from build123d import *

# Parameters (mm, degrees)
SKETCH1_W           = 40
SKETCH1_H           = 28.8
BOSS_EXTRUDE1_DEPTH = 11
CHAMFER2_SIZE       = 8
CHAMFER2_SIZE2      = 18
SKETCH10_W          = 13.5
SKETCH10_H          = 18.8
CUT_EXTRUDE7_DEPTH  = 6
FILLET1_R           = 1.5
SKETCH11_W          = 40
SKETCH11_H          = 3
CUT_EXTRUDE8_DEPTH  = 8
CUT_EXTRUDE9_DEPTH  = 18.8
CUT_EXTRUDE10_DEPTH = 11
CUT_EXTRUDE2_DEPTH  = 30
SKETCH2_R           = 1.65
CUT_EXTRUDE1_DEPTH  = 12
CUT_EXTRUDE4_DEPTH  = 9
SKETCH15_R          = 3.25
CUT_EXTRUDE12_DEPTH = 1
CUT_EXTRUDE13_DEPTH = 6
CHAMFER4_SIZE       = 3
CHAMFER4_SIZE2      = 5
CHAMFER5_SIZE       = 5
CHAMFER5_SIZE2      = 3
CUT_EXTRUDE11_DEPTH = 9.4
CHAMFER8_SIZE       = 1


with BuildPart() as part:
    # Sketch1 → Boss-Extrude1 (new body)
    with BuildSketch(Plane.XY):
        with Locations((0, 14.4)):
            Rectangle(SKETCH1_W, SKETCH1_H)
    extrude(amount=BOSS_EXTRUDE1_DEPTH)

    # Chamfer2
    chamfer2_edges = [part.edges().sort_by_distance(p)[0] for p in [
        (0, 28.8, 11),
    ]]
    chamfer2_side = [part.faces().sort_by_distance(p)[0] for p in [
        (0, 28.8, 5.5),
    ]]
    chamfer(chamfer2_edges, length=CHAMFER2_SIZE, length2=CHAMFER2_SIZE2, reference=chamfer2_side[0])

    # Sketch10 → Cut-Extrude7 (cut)
    with BuildSketch(Plane.XY.offset(11)):
        with Locations((-13.25, 19.4)):
            Rectangle(SKETCH10_W, SKETCH10_H)
        with Locations((13.25, 19.4)):
            Rectangle(SKETCH10_W, SKETCH10_H)
    extrude(amount=-CUT_EXTRUDE7_DEPTH, mode=Mode.SUBTRACT)

    # Fillet1
    fillet1_edges = [part.edges().sort_by_distance(p)[0] for p in [
        (-13.25, 10, 5),
        (13.25, 10, 5),
    ]]
    fillet(fillet1_edges, radius=FILLET1_R)

    # Sketch11 → Cut-Extrude8 (cut)
    with BuildSketch(Plane.XY.offset(11)):
        with Locations((0, 1.5)):
            Rectangle(SKETCH11_W, SKETCH11_H)
    extrude(amount=-CUT_EXTRUDE8_DEPTH, mode=Mode.SUBTRACT)

    # Sketch12 → Cut-Extrude9 (cut)
    with BuildSketch(Plane(origin=(0, 28.8, 0), x_dir=(1, 0, 0), z_dir=(0, 1, 0))):
        with BuildLine():
            Line((-4.25, -8), (-4.25, -11))
            Line((-4.25, -11), (-10.75, -11))
            Line((-10.75, -11), (-10.75, -8))
            ThreePointArc((-10.75, -8), (-7.5, -4.75), (-4.25, -8))
        make_face()
    cut_extrude9 = extrude(amount=-CUT_EXTRUDE9_DEPTH, mode=Mode.SUBTRACT)

    # Sketch13 → Cut-Extrude10 (cut, through all)
    with BuildSketch(Plane(origin=(0, 10, 0), x_dir=(1, 0, 0), z_dir=(0, 1, 0))):
        with BuildLine():
            Line((-9.15, -8), (-9.15, -11))
            Line((-9.15, -11), (-5.85, -11))
            Line((-5.85, -11), (-5.85, -8))
            ThreePointArc((-5.85, -8), (-7.5, -6.35), (-9.15, -8))
        make_face()
    cut_extrude10 = extrude(amount=-CUT_EXTRUDE10_DEPTH, mode=Mode.SUBTRACT)

    # Sketch3 → Cut-Extrude2 (cut)
    with BuildSketch(Plane.XZ):
        with BuildLine():
            Line((-3.25, 8), (-3.25, 11))
            Line((-3.25, 11), (3.25, 11))
            Line((3.25, 11), (3.25, 8))
            ThreePointArc((3.25, 8), (0, 4.75), (-3.25, 8))
        make_face()
    extrude(amount=-CUT_EXTRUDE2_DEPTH, mode=Mode.SUBTRACT)

    # Sketch2 → Cut-Extrude1 (cut, through all)
    with BuildSketch(Plane.XY.offset(11)):
        with Locations((-12.5, 2.9)):
            Circle(SKETCH2_R)
        with Locations((12.5, 2.9)):
            Circle(SKETCH2_R)
        with Locations((12.5, 25.9)):
            Circle(SKETCH2_R)
        with Locations((-12.5, 25.9)):
            Circle(SKETCH2_R)
    extrude(amount=-CUT_EXTRUDE1_DEPTH, mode=Mode.SUBTRACT)

    # Sketch5 → Cut-Extrude4 (cut)
    with BuildSketch(Plane.XY.offset(11)):
        Polygon((-13.825512835, 29.376278709), (-11.142302486, 29.376278709), (-9.151427839, 25.880054666), (-10.842987085, 22.990078775), (-14.191559246, 23.010024109), (-15.848572161, 25.919945334), align=None)
        Polygon((11.142302486, 29.376278709), (13.825512835, 29.376278709), (15.848572161, 25.919945334), (14.191559246, 23.010024109), (10.842987085, 22.990078775), (9.151427839, 25.880054666), align=None)
    extrude(amount=-CUT_EXTRUDE4_DEPTH, mode=Mode.SUBTRACT)

    # Sketch15 → Cut-Extrude12 (cut)
    with BuildSketch(Plane(origin=(0, 10, 0), x_dir=(1, 0, 0), z_dir=(0, 1, 0))):
        with Locations((-7.5, -8)):
            Circle(SKETCH15_R)
    cut_extrude12 = extrude(amount=-CUT_EXTRUDE12_DEPTH, mode=Mode.SUBTRACT)

    # Sketch16 → Cut-Extrude13 (cut, through all)
    with BuildSketch(Plane.XY.offset(5)):
        with BuildLine():
            Line((-15, 14), (-15, 19))
            ThreePointArc((-15, 19), (-12.5, 21.5), (-10, 19))
            Line((-10, 19), (-10, 14))
            ThreePointArc((-10, 14), (-12.5, 11.5), (-15, 14))
        make_face()
    cut_extrude13 = extrude(amount=-CUT_EXTRUDE13_DEPTH, mode=Mode.SUBTRACT)

    # Mirror1: Cut-Extrude9, Cut-Extrude10, Cut-Extrude12, Cut-Extrude13 across plane
    add(cut_extrude9.mirror(Plane(origin=(0, 0, 0), x_dir=(0, 0, 1), z_dir=(1, 0, 0))), mode=Mode.SUBTRACT)
    add(cut_extrude10.mirror(Plane(origin=(0, 0, 0), x_dir=(0, 0, 1), z_dir=(1, 0, 0))), mode=Mode.SUBTRACT)
    add(cut_extrude12.mirror(Plane(origin=(0, 0, 0), x_dir=(0, 0, 1), z_dir=(1, 0, 0))), mode=Mode.SUBTRACT)
    add(cut_extrude13.mirror(Plane(origin=(0, 0, 0), x_dir=(0, 0, 1), z_dir=(1, 0, 0))), mode=Mode.SUBTRACT)

    # Chamfer4
    chamfer4_edges = [part.edges().sort_by_distance(p)[0] for p in [
        (20, 28.8, 1.5),
    ]]
    chamfer4_side = [part.faces().sort_by_distance(p)[0] for p in [
        (20, 12.613389716, 3.722385656),
    ]]
    chamfer(chamfer4_edges, length=CHAMFER4_SIZE, length2=CHAMFER4_SIZE2, reference=chamfer4_side[0])

    # Chamfer5
    chamfer5_edges = [part.edges().sort_by_distance(p)[0] for p in [
        (-20, 28.8, 1.5),
    ]]
    chamfer5_side = [part.faces().sort_by_distance(p)[0] for p in [
        (-2.670324549, 28.8, 1.43187018),
    ]]
    chamfer(chamfer5_edges, length=CHAMFER5_SIZE, length2=CHAMFER5_SIZE2, reference=chamfer5_side[0])

    # Sketch14 → Cut-Extrude11 (cut)
    with BuildSketch(Plane.XY.offset(11)):
        Polygon((-9.151368439, 2.9), (-10.825684219, 5.8), (-14.174315781, 5.8), (-15.848631561, 2.9), (-14.174315781, 0), (-10.825684219, 0), align=None)
        Polygon((15.848631561, 2.9), (14.174315781, 5.8), (10.825684219, 5.8), (9.151368439, 2.9), (10.825684219, 0), (14.174315781, 0), align=None)
    extrude(amount=-CUT_EXTRUDE11_DEPTH, mode=Mode.SUBTRACT)

    # Chamfer8
    chamfer8_edges = [part.edges().sort_by_distance(p)[0] for p in [
        (20, 0, 1.5),
        (-20, 0, 1.5),
    ]]
    chamfer(chamfer8_edges, length=CHAMFER8_SIZE)


solid = part.part
Geometry: final body of the model. Coordinates: model frame, mm. A direction names the side the tool comes from. Give positions to 0.01 mm unless a question says otherwise; leave off trailing zeros. Order: outer loops, then holes, each group sorted by start corner. A loop starts at its lowest first (then second) coordinate and runs counter-clockwise, first axis right, second up. Notation, with made-up numbers: (-38, 40) -> (7, 40) arc R13 cw to (7, 65) -> close; hole circle Ø8 at (-35, -10). An arc over 180 degrees is marked (long way). Answer as a JSON object with one key per item and string values.
Q1. Section A-A (y = 20.75). Output: boundary loops of the cut face in (x, z), plus the area to 3 significant figures.
Entries:
{"outline": "(-20, 0) -> (-14.29, 0) -> (-14.29, 5) -> (-20, 5) -> close; (-10.71, 0) -> (10.71, 0) -> (10.71, 5) -> (8.75, 5) arc R3.25 cw to (4.58, 6.58) -> (2.92, 6.58) arc R3.25 cw to (-2.92, 6.58) -> (-4.58, 6.58) arc R3.25 cw to (-8.75, 5) -> (-10.71, 5) -> close; (14.29, 0) -> (20, 0) -> (20, 5) -> (14.29, 5) -> close", "area": "172 mm^2"}
Q2. Section B-B (x = 7.5). Output: boundary loops of the cut face in (y, z), plus the area to 3 significant figures.
Entries:
{"outline": "(0, 0) -> (28.8, 0) -> (28.8, 3) -> (24.86, 4.75) -> (9, 4.75) -> (9, 6.35) -> (3, 6.35) -> (3, 3) -> (0, 3) -> close", "area": "138 mm^2"}
Q3. Draft query along Y for faces 1 (the flat face through (19.5, 0.5, 1.5)), 2 (the cylindrical face through (-7.46, 6.04, 6.35)), 3 (the flat face through (15, 16, 3)). Return one class per face: released by +Y, released by -Y, zero draft, split by the parting line, or undercut.
Entries:
{"face 1": "released by -Y", "face 2": "zero draft", "face 3": "undercut"}
Q4. First-contact query: pin 1 (2.5 mm diameter, centred on x = -16.5, y = 1.5, fed in from +Z); pin 2 (3.5 mm diameter, centred on x = -12, z = 4.5, fed in from -Y); pin 3 (1.7 mm diameter, centred on x = -13.5, y = 2.5, fed in from +Z). Flat tips, straight axial feed; report the tip coordinate or a pass-through.
Entries:
{"pin 1": "stops at z = 3", "pin 2": "stops at y = 4.8", "pin 3": "stops at z = 1.6"}
Q5. Section C-C (y = 6.25). Output: boundary loops of the cut face in (x, z), plus the area to 3 significant figures.
Entries:
{"outline": "(-20, 0) -> (20, 0) -> (20, 11) -> (9.15, 11) -> (9.15, 8) arc R1.65 cw to (5.85, 8) -> (5.85, 11) -> (3.25, 11) -> (3.25, 8) arc R3.25 cw to (-3.25, 8) -> (-3.25, 11) -> (-5.85, 11) -> (-5.85, 8) arc R1.65 cw to (-9.15, 8) -> (-9.15, 11) -> (-20, 11) -> close", "area": "376 mm^2"}
Q6. Access query for faces 4 (the flat face through (14, 10, 9)), 5 (the flat face through (5.85, 7, 10)), 6 (the flat face through (15, 1.43, 2.31)), 7 (the flat face through (-18, 3, 7)). Directions: +Z, -Z, +X, -X, +Y, -Y. A direction counts if a zero-diameter tool reaches every point of the face in a straight line with its end or side. Return the directions, or none.
Entries:
{"face 4": "+Z, +X, +Y", "face 5": "+Z, +Y, -Y", "face 6": "+Z", "face 7": "+Z, +X, -X, -Y"}
Q7. Material intervals for probe 1 along Y at (x, z) = (12.5, 1.05); probe 2 along X at (y, z) = (11.75, 8.25); probe 3 along X at (y, z) = (12.75, 2), sorted ascending.
Entries:
{"probe 1": "y = 0 to 1.25, 4.55 to 11.5, 21.5 to 24.25, 27.55 to 28.8", "probe 2": "x = -4.25 to -3.25, 3.25 to 4.25", "probe 3": "x = -20 to -14.67, -10.33 to 10.33, 14.67 to 20"}
Q8. Section D-D (y = 2.25). Output: boundary loops of the cut face in (x, z).
Entries:
{"outline": "(-20, 0) -> (-14.02, 0) -> (-14.02, 1.6) -> (-15.47, 1.6) -> (-15.47, 3) -> (-20, 3) -> close; (-10.98, 0) -> (10.98, 0) -> (10.98, 1.6) -> (9.53, 1.6) -> (9.53, 3) -> (-9.53, 3) -> (-9.53, 1.6) -> (-10.98, 1.6) -> close; (14.02, 0) -> (20, 0) -> (20, 3) -> (15.47, 3) -> (15.47, 1.6) -> (14.02, 1.6) -> close"}
